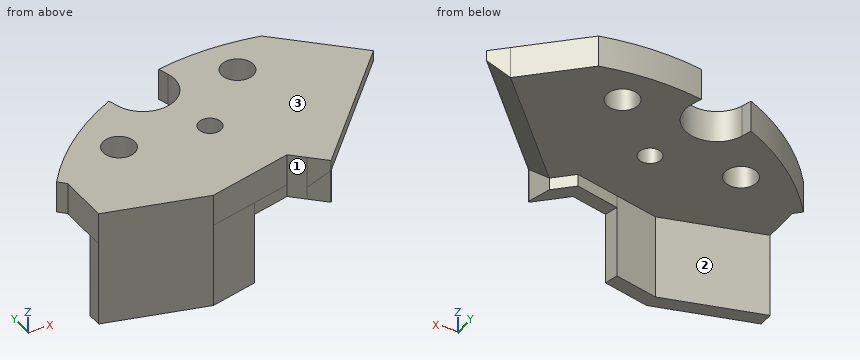
```python
from build123d import *

# Parameters (mm, degrees)
ESTRUSIONE_ESTRUSIONE1_DEPTH = 9
ESTRUSIONE_SOTTILE1_DEPTH    = 3
ESTRUSIONE_ESTRUSIONE2_DEPTH = 3.5
SCHIZZO4_W                   = 9.5
SCHIZZO4_H                   = 0.5
ESTRUSIONE_ESTRUSIONE3_DEPTH = 0.1
ESTRUSIONE_ESTRUSIONE4_DEPTH = 24
SCHIZZO6_R                   = 4.5
SCHIZZO6_R_2                 = 3.2
TAGLIO_ESTRUSIONE1_DEPTH     = 81.740882068


with BuildPart() as part:
    # Schizzo1 → Estrusione-Estrusione1 (new body)
    with BuildSketch(Plane.XY):
        with BuildLine():
            Line((-3.647686021, 3.419705644), (0, 0))
            Line((0, 0), (32.145233057, 34.288248595))
            Line((32.145233057, 34.288248595), (16.145233057, 49.288248595))
            ThreePointArc((16.145233057, 49.288248595), (1.884416467, 51.07583724), (-12.447686021, 50.000104337))
            Line((-12.447686021, 50.000104337), (-11.562006013, 47.13559635))
            ThreePointArc((-11.562006013, 47.13559635), (-17.502963658, 35.876553995), (-28.762006013, 41.81751164))
            Line((-28.762006013, 41.81751164), (-29.647686021, 44.682019626))
            ThreePointArc((-29.647686021, 44.682019626), (-45.119453561, 35.169318817), (-57.724052903, 22.09296065))
            Line((-57.724052903, 22.09296065), (-55.714897525, 20.102116027))
            Line((-55.714897525, 20.102116027), (-55.647686021, 5.419705644))
            Line((-55.647686021, 5.419705644), (-27.647686021, -2.080294356))
            Line((-27.647686021, -2.080294356), (-3.647686021, 3.419705644))
        make_face()
    extrude(amount=ESTRUSIONE_ESTRUSIONE1_DEPTH)


with BuildPart() as body_2:
    # Schizzo2 → Estrusione-Sottile1 (new body)
    with BuildSketch(Plane.XY.offset(9)):
        Polygon((36.522456282, 30.184601821), (4.377223225, -4.103646773), (4.340746365, -4.069449717), (36.485979422, 30.218798878), align=None)
    extrude(amount=-ESTRUSIONE_SOTTILE1_DEPTH)


    add(part.part)  # loft1 joins it to this body
    # loft from a face of the part (loft1)
    loft([body_2.faces().sort_by_distance((20.413362893, 13.07467458, 7.5))[0], body_2.faces().sort_by_distance((16.072616529, 17.144124297, 4.5))[0]])

    # Schizzo3 → Estrusione-Estrusione2 (add)
    with BuildSketch(Plane(origin=(0, 0, 0), x_dir=(-1, 0, 0), z_dir=(0, 0, -1))):
        Polygon((0, 0), (3.647686021, 3.419705644), (14.243498137, 0.991498701), (15.137002762, 4.890427975), (2.465482621, 7.794318007), (-2.735764516, 2.918148817), align=None)
    extrude(amount=ESTRUSIONE_ESTRUSIONE2_DEPTH)

    # Schizzo4 → Estrusione-Estrusione3 (add)
    with BuildSketch(Plane(origin=(4.377223225, -4.103646773, 0), x_dir=(0, 0, -1), z_dir=(0.7295372041400824, -0.6839411288813327, 0))):
        with Locations((-1.25, 0.25)):
            Rectangle(SCHIZZO4_W, SCHIZZO4_H)
    extrude(amount=-ESTRUSIONE_ESTRUSIONE3_DEPTH)

    # loft from a face of the part (loft3)
    loft([body_2.faces().sort_by_distance((4.475254787, -3.852868359, 1.224789916))[0], body_2.faces().sort_by_distance((1.367882258, 1.459074408, -1.75))[0]])

    # Schizzo5 → Estrusione-Estrusione4 (add)
    with BuildSketch(Plane(origin=(0, 0, 0), x_dir=(-1, 0, 0), z_dir=(0, 0, -1))):
        Polygon((14.243498137, 0.991498701), (27.647686021, -2.080294356), (55.647686021, 5.419705644), (55.666665545, 9.565798886), (27.686647069, 2.07115108), (15.137002762, 4.890427975), align=None)
    extrude(amount=ESTRUSIONE_ESTRUSIONE4_DEPTH)

    # Schizzo6 → Taglio-Estrusione1 (cut, through all)
    with BuildSketch(Plane(origin=(0, 0, 0), x_dir=(-1, 0, 0), z_dir=(0, 0, -1))):
        with Locations((-3.975977763, 40.135945247)):
            Circle(SCHIZZO6_R)
        with Locations((13.659623442, 23.345827018)):
            Circle(SCHIZZO6_R_2)
        with Locations((37.256730628, 26.89249206)):
            Circle(SCHIZZO6_R)
    extrude(amount=-TAGLIO_ESTRUSIONE1_DEPTH, mode=Mode.SUBTRACT)


solid = body_2.part
```
Geometry check sheet. Reference: the model listing, model coordinates, mm. Face numbers are marked on the shaded views. A direction names the side the tool comes from. Round coordinates to 2 decimals unless told otherwise and drop trailing zeros. Loops run counter-clockwise (first coordinate to the right, second up) from the corner with the lowest first, then second, coordinate; pieces in that order, holes last. Notation, with made-up numbers: M -35.75,23.25 L -13.75,23.25 A10 cw -13.75,34.25 Z; hole C 23.25,5 d10. An arc over 180 degrees is marked long. Return JSON: item names as keys, results as strings. Group by question number.
(1) Set-up check for the marked faces 1, 2 and 3: record each of +Z, -Z, +X, -X, +Y, -Y from which the full face is reachable in a straight line by a thin tool's end or side.
(2) Section check B-B, the plane z = -16.5. Enter the section's corners in (x, y).
(3) Scan lines: line 1 along X through (y, z) = (23.5, 1.5); line 2 along Z through (x, y) = (0, 46); line 3 along X through (y, z) = (30.5, 6). Record each from-to range of solid material in increasing order. Write a range as [from, to].
(4) Go/stop test with flat-tipped pins: pin 1 (3 mm diameter, centred on x = 9, z = 0, fed in from +Y); pin 2 (3 mm diameter, centred on x = -16, z = 3, fed in from +Y); pin 3 (6 mm diameter, centred on x = -12, y = 27, fed in from -Z). Record where each tip stops, or that it passes through.
(5) Section check C-C, the plane z = 1. Give the number of separate pieces and of enclosed holes in the cut face, and give its area (3 significant figures).
(6) Section check A-A, the plane x = -48.5. Enter the section's corners in (y, z).
Data:
{
 "1": {"face 1": "+Z, -Z, -Y", "face 2": "-Z, +Y", "face 3": "+Z, +X, -X, +Y, -Y"},
 "2": {"outline": "M -55.67,9.57 L -55.65,5.42 L -27.65,-2.08 L -14.24,0.99 L -15.14,4.89 L -27.69,2.07 Z"},
 "3": {"line 1": "[-56.65, -40.21], [-34.3, -16.86], [-10.46, 24.07]", "line 2": "[0, 9]", "line 3": "[-50.38, -39.95], [-34.57, 36.19]"},
 "4": {"pin 1": "y = 50.72", "pin 2": "y = 37.48", "pin 3": "z = 0"},
 "5": {"separate pieces": "1", "enclosed holes": "3", "area": "2,970 mm²"},
 "6": {"outline": "M 3.51,-24 L 7.65,-24 L 7.65,0 L 32.27,0 L 32.27,9 L 3.51,9 Z"}
}
